Can you work these out from the model? Positions are in its coordinate system, mm. Give positions to 0.01 mm unless a question says otherwise; leave off trailing zeros. Loops run counter-clockwise (first coordinate to the right, second up) from the corner with the lowest first, then second, coordinate; pieces in that order, holes last. Notation, with made-up numbers: M 65.25,63.5 L 95.25,63.5 A25 cw 95.25,89.5 Z; hole C -37,-20 d6. An arc over 180 degrees is marked long. Answer as a JSON object with one key per item and string values.
```python
from build123d import *

# Parameters (mm, degrees)
F0_R     = 6.731
F1_DEPTH = 9.525


with BuildPart() as f1:
    # F0 (on Top) → F1 (new body)
    with BuildSketch(Plane.XY):
        with BuildLine():
            ThreePointArc((82.55, -88.9), (87.040128, -87.040128), (88.9, -82.55))
            Line((88.9, -82.55), (88.9, 82.55))
            ThreePointArc((88.9, 82.55), (87.040128, 87.040128), (82.55, 88.9))
            Line((82.55, 88.9), (-88.9, 88.9))
            Line((-88.9, 88.9), (-88.9, -88.9))
            Line((-88.9, -88.9), (82.55, -88.9))
        make_face()
        with Locations((23.506227, -49.9999)):
            Circle(F0_R, mode=Mode.SUBTRACT)
        with Locations((63.506147, -49.9999)):
            Circle(F0_R, mode=Mode.SUBTRACT)
        with Locations((23.506227, 49.9999)):
            Circle(F0_R, mode=Mode.SUBTRACT)
        with Locations((63.506147, 49.9999)):
            Circle(F0_R, mode=Mode.SUBTRACT)
    extrude(amount=F1_DEPTH)


solid = f1.part
```
1) If we mould it in two halves opening along Y, with no side actions, what happens to faces 1 (the flat face through (-1, 1, 9.525)), 2 (the cylindrical face through (27.12, -44.32, 4.7)), 3 (the cylindrical face through (86.99, -87.09, 4.7))? For each: +Y half, -Y half, draft (parallel to the pull), parting line (faces both ways), or undercut.
Answer list:
{"face 1": "draft", "face 2": "undercut", "face 3": "-Y half"}
2) Suppose I cut it at B-B, the plane z = 3.5. Write out the boundary of the cut face in (x, y).
Answer list:
{"outline": "M -88.9,-88.9 L 82.55,-88.9 A6.35 ccw 88.9,-82.55 L 88.9,82.55 A6.35 ccw 82.55,88.9 L -88.9,88.9 Z; hole C 23.51,-50 d13.46; hole C 23.51,50 d13.46; hole C 63.51,-50 d13.46; hole C 63.51,50 d13.46"}
3) Will this pin go through, and if not, where does the flat tip stop? pin 1 Ø21.5 at (x, y) = (63.51, 50) entering from +Z (3 decimals).
Answer list:
{"pin 1": "z = 9.525"}
4) Please list where these lines run through material, in increasing order: line 1 along Y through (x, z) = (25.5, 8.25); line 2 along X through (y, z) = (47.5, 3); line 3 along Y through (x, z) = (69, 7). Write a range as from..to.
Answer list:
{"line 1": "-88.9..-56.43, -43.57..43.57, 56.43..88.9", "line 2": "-88.9..17.26, 29.76..57.26, 69.76..88.9", "line 3": "-88.9..-53.89, -46.11..46.11, 53.89..88.9"}
5) Suppose I cut it at C-C, the plane x = 28. Write out the boundary of the cut face in (y, z) (3 decimals), and give its area (3 significant figures).
Answer list:
{"outline": "M -88.9,0 L -55.011,0 L -55.011,9.525 L -88.9,9.525 Z; M -44.989,0 L 44.989,0 L 44.989,9.525 L -44.989,9.525 Z; M 55.011,0 L 88.9,0 L 88.9,9.525 L 55.011,9.525 Z", "area": "1,500 mm^2"}
6) Suppose I cut it at A-A, the plane x = 62. Write out the boundary of the cut face in (y, z) (3 decimals), and give its area (3 significant figures).
Answer list:
{"outline": "M -88.9,0 L -56.56,0 L -56.56,9.525 L -88.9,9.525 Z; M -43.44,0 L 43.44,0 L 43.44,9.525 L -43.44,9.525 Z; M 56.56,0 L 88.9,0 L 88.9,9.525 L 56.56,9.525 Z", "area": "1,440 mm^2"}
